The model under review builds one solid part; all positions refer to its coordinate system, in mm. A direction names the side the tool comes from. Round coordinates to 2 decimals unless told otherwise and drop trailing zeros. Write each loop counter-clockwise with the first axis right and the second up, starting at its lowest first coordinate (ties: lowest second). Pieces come first, ordered by that corner, then holes.
Item 1: Add section A-A (y = 24). Give the boundary of the cut face in (x, z), plus the area to 3 significant figures.
Item 2: Clearance check with flat-ended pins moving along their axes: pin 1 Ø4 at (y, z) = (3.5, 2.5) entering from -X; pin 2 Ø5 at (y, z) = (21.5, -8.5) entering from -X; pin 3 Ø5 at (y, z) = (8.5, -7.5) entering from +X. State where each tip first meets the part, or that it passes through.
Item 3: To check wall thickness, follow L1, parallel to Z at x = 0, y = 19; L2, parallel to Y at x = 3.75, z = 9.5; L3, parallel to Z at x = 3.25, y = 14.75. State the ranges of each line that lie inside material, in increasing order.
Item 4: Draft analysis for pull direction Y (two halves, no side actions). For faces 1 (the face through (9.54, 25.84, 3)), 2 (the face through (10, 14.9, 3.2)), state which applies: +Y half, -Y half, draft (parallel to the pull), parting line (faces both ways), or undercut.
Item 5: Machinability: for faces 3 (the face through (10, 28, 3.2)), 4 (the face through (9.54, 4.14, 3)), which of the approach directions +Z, -Z, +X, -X, +Y, -Y give a long, thin tool a straight path to every point of the face, cutting with its end or side? Answer none if there is none.
```python
from build123d import *


with BuildPart() as f2:
    # F2: sweep along a path in F0
    with BuildLine(Plane.XZ) as f2_path:
        CenterArc((0, 0), 6, 0, 360)
    # F1 (on Right) → F2 (sweep)
    with BuildSketch(Plane.YZ):
        Polygon((0, 10), (0, 6), (30, 6), (30, 10), (29.5, 10.5), (26.5, 10.5), (26.5, 10), (25.2, 10), (25.2, 10.5), (15, 10.5), (4.8, 10.5), (4.8, 10), (3.5, 10), (3.5, 10.5), (0.5, 10.5), align=None)
    sweep(path=f2_path.line)


solid = f2.part
```
Numbers:
1. outline: circle Ø21 at (0, 0); hole circle Ø12 at (0, 0)
1. area: 233 mm2
2. pin 1: stops at x = -10.49
2. pin 2: stops at x = -8.62
2. pin 3: stops at x = 9.23
3. L1: z = -10.5 to -6, 6 to 10.5
3. L2: y = 0.21 to 3.5, 4.8 to 25.2, 26.5 to 29.79
3. L3: z = -9.98 to -5.04, 5.04 to 9.98
4. face 1: undercut
4. face 2: draft
5. face 3: +Y, -Y
5. face 4: none
